The drawing under review shows one solid part. Ordinate dimensions are in mm from its lowest x, y, z. A direction names the side the tool comes from. Round coordinates to 2 decimals unless told otherwise and drop trailing zeros. Order: outer loops, then holes, each group sorted by start corner. A loop starts at its lowest first (then second) coordinate and runs counter-clockwise, first axis right, second up. Notation, with made-up numbers: (51, 27.25) -> (69, 27.25) arc R23 ccw to (69, 53.25) -> close; hole circle Ø9 at (42, 22.25). An arc over 180 degrees is marked (long way). Use a Markdown table: item, result. Add a question column.
1) Draft analysis for pull direction X (two halves, no side actions). For the marked faces 1, 2 and 3, state which applies: pulls with the +X half, pulls with the -X half, needs draft (parallel to the pull), parting line crosses it, or undercut.
2) Consider section D-D (y = 5.75). State the section outline as (x, z) points, plus the area to 3 significant figures.
3) Wall thickness on line 1 along Z through (x, y) = (33, 5.25); line 2 along X through (y, z) = (2.5, 11.5); line 3 along Z through (x, y) = (22, 8.75): over which ranges is each line inside the solid? List them lowest first. Write a range as [from, to].
4) Consider section A-A (z = 10). State the section outline as (x, y) points, plus the area to 3 significant figures.
5) Machinability: for the marked faces 4 and 5, which of the approach directions +Z, -Z, +X, -X, +Y, -Y give a long, thin tool a straight path to every point of the face, cutting with its end or side? Answer none if there is none.
6) Consider section B-B (y = 2.5). State the section outline as (x, z) points.
7) Consider section C-C (x = 7). State the section outline as (y, z) points, plus the area to 3 significant figures.
8) Clearance check with a flat-ended pin moving along its axis: P1, Ø4, axis at x = 22, y = 8, coming from the -Z side. State where the tip first meets the part, or that it passes through.
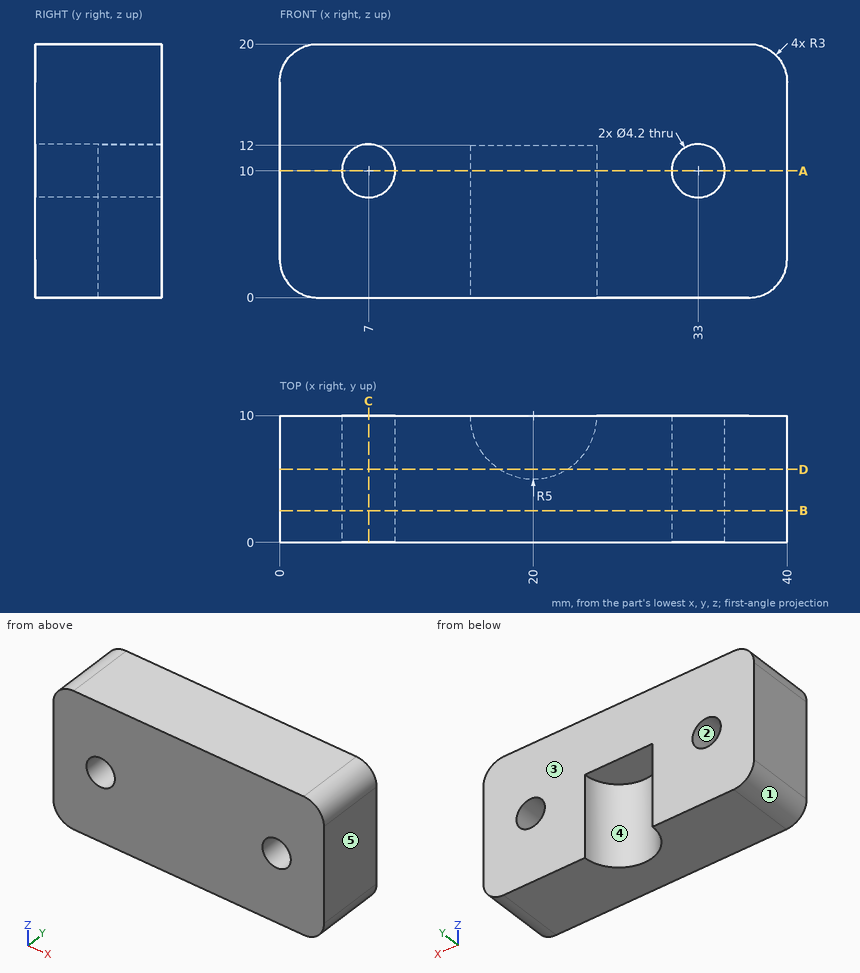
Results list:
| question | item | result |
|---|---|---|
| 1 | face 1 | pulls with the -X half |
| 1 | face 2 | undercut |
| 1 | face 3 | needs draft |
| 2 | outline | (0, 3) arc R3 ccw to (3, 0) -> (17.37, 0) -> (17.37, 12) -> (22.63, 12) -> (22.63, 0) -> (37, 0) arc R3 ccw to (40, 3) -> (40, 17) arc R3 ccw to (37, 20) -> (3, 20) arc R3 ccw to (0, 17) -> close; hole circle Ø4.2 at (7, 10); hole circle Ø4.2 at (33, 10) |
| 2 | area | 701 mm2 |
| 3 | line 1 | [0, 7.9], [12.1, 20] |
| 3 | line 2 | [0, 5.53], [8.47, 31.53], [34.47, 40] |
| 3 | line 3 | [12, 20] |
| 4 | outline | (0, 0) -> (4.9, 0) -> (4.9, 10) -> (0, 10) -> close; (9.1, 0) -> (30.9, 0) -> (30.9, 10) -> (25, 10) arc R5 cw to (15, 10) -> (9.1, 10) -> close; (35.1, 0) -> (40, 0) -> (40, 10) -> (35.1, 10) -> close |
| 4 | area | 277 mm2 |
| 5 | face 4 | -Z, +Y |
| 5 | face 5 | +Z, -Z, +X, +Y, -Y |
| 6 | outline | (0, 3) arc R3 ccw to (3, 0) -> (37, 0) arc R3 ccw to (40, 3) -> (40, 17) arc R3 ccw to (37, 20) -> (3, 20) arc R3 ccw to (0, 17) -> close; hole circle Ø4.2 at (7, 10); hole circle Ø4.2 at (33, 10) |
| 7 | outline | (0, 0) -> (10, 0) -> (10, 7.9) -> (0, 7.9) -> close; (0, 12.1) -> (10, 12.1) -> (10, 20) -> (0, 20) -> close |
| 7 | area | 158 mm2 |
| 8 | P1 | z = 12 |
